Part model, mm, in its own coordinate system. Face numbers are marked on the shaded views. A direction names the side the tool comes from. Give positions to 0.01 mm unless a question says otherwise; leave off trailing zeros. Write each loop counter-clockwise with the first axis right and the second up, starting at its lowest first coordinate (ties: lowest second). Pieces come first, ordered by that corner, then holes.
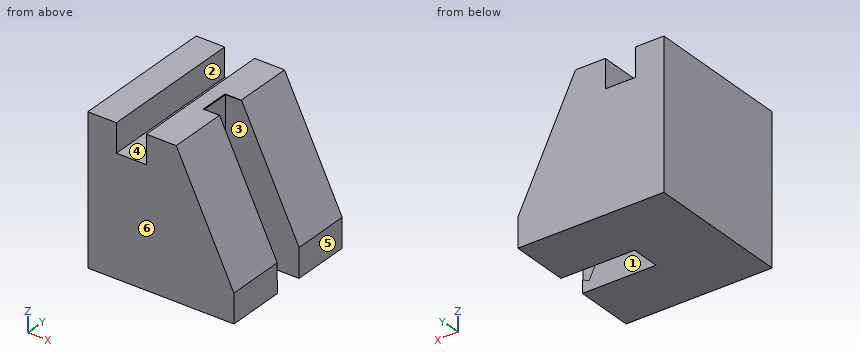
from build123d import *

# Parameters (mm, degrees)
F1_DEPTH = 100
F2_W     = 20
F2_H     = 89.6053736129
F3_DEPTH = 10
F4_DEPTH = 10
F5_DEPTH = 10
F6_W     = 50.2936672419
F6_H     = 19.8401175439
F7_DEPTH = 100


with BuildPart() as f1:
    # F0 (on Front) → F1 (new body)
    with BuildSketch(Plane.XZ):
        Polygon((-55.1563166082, 75.4929259419), (-74.7038125992, 75.4929259419), (-74.7038125992, -24.8185619712), (25.1119807363, -24.8185619712), (25.1119807363, -4.9872435629), (-14.2842791975, 75.4929259419), (-34.7202979028, 75.4929259419), (-34.7202979028, 55.9454262257), (-55.1563166082, 55.9454262257), align=None)
    extrude(amount=F1_DEPTH)

    # F2 (on face) → F3 (cut)
    with BuildSketch(Plane(origin=(18.2883118785, 0, 8.9524052067), x_dir=(0, 1, 0), z_dir=(0.8981623117, 0, 0.4396640329))):
        with Locations((-50, 29.2824978739)):
            Rectangle(F2_W, F2_H)
    extrude(amount=-F3_DEPTH, mode=Mode.SUBTRACT)

    # F4 (cut): a face of the model
    f4_faces = [f1.faces().sort_by_distance(p)[0] for p in [
        (-18.775090756, -50, 73.2946057774),
    ]]
    extrude(f4_faces, amount=-F4_DEPTH, mode=Mode.SUBTRACT)

    # F5 (cut): a face of the model
    f5_faces = [f1.faces().sort_by_distance(p)[0] for p in [
        (20.6211691778, -50, -7.1855637275),
    ]]
    extrude(f5_faces, amount=-F5_DEPTH, mode=Mode.SUBTRACT)

    # F6 (on face) → F7 (cut)
    with BuildSketch(Plane(origin=(0, 0, -24.8185619712), x_dir=(1, 0, 0), z_dir=(0, 0, -1))):
        with Locations((-0.0348528847, 49.7383717448)):
            Rectangle(F6_W, F6_H)
    extrude(amount=-F7_DEPTH, mode=Mode.SUBTRACT)


solid = f1.part
1) Drill centre lines: L1, parallel to Y at x = 15, z = -16.5; L2, parallel to Y at x = 13, z = 16.5; L3, parallel to Z at x = -50, y = -27. Where is each one in solid material? Low to high.
Check result:
L1: y = -100 to -59.66, -39.82 to 0
L2: y = -100 to -60, -39.82 to 0
L3: z = -24.82 to 55.95
2) Saw through at C-C (z = -1). Write the cut outline in (x, y).
Check result:
outline: (-74.7, -100) - (23.16, -100) - (23.16, -60) - (12.03, -60) - (12.03, -59.66) - (-25.18, -59.66) - (-25.18, -39.82) - (23.16, -39.82) - (23.16, 0) - (-74.7, 0) - close
3) Mould opens along X. For the marked faces 4, 5 and 6 say: +X half, -X half, draft (parallel to the pull), parting line (faces both ways), or undercut.
Check result:
face 4: undercut
face 5: +X half
face 6: draft
4) 3-axis set-ups, long thin cutter, end or side, ignore diameter. For the marked faces 1, 2 and 3: which of +Z, -Z, +X, -X, +Y, -Y reach the whole face in a straight line?
Check result:
face 1: +Z, -Z, +X
face 2: +Z, +Y, -Y
face 3: -Z, +X
5) Saw through at B-B (y = -9.5). Write the cut outline in (x, z), and give its area (3 significant figures).
Check result:
outline: (-74.7, -24.82) - (25.11, -24.82) - (25.11, -4.99) - (-14.28, 75.49) - (-34.72, 75.49) - (-34.72, 55.95) - (-55.16, 55.95) - (-55.16, 75.49) - (-74.7, 75.49) - close
area: 8,030 mm2
6) Saw through at A-A (x = -19.5). Write the cut outline in (y, z).
Check result:
outline: (-100, -24.82) - (-59.66, -24.82) - (-59.66, 63.4) - (-60, 63.4) - (-60, 75.49) - (-100, 75.49) - close; (-40, 75.18) - (-39.82, 75.18) - (-39.82, -24.82) - (0, -24.82) - (0, 75.49) - (-40, 75.49) - close
7) Saw through at D-D (x = -44). Write the cut outline in (y, z).
Check result:
outline: (-100, -24.82) - (0, -24.82) - (0, 55.95) - (-100, 55.95) - close
8) Flat gauge pins, fed straight in: P1, Ø10, axis at y = -51.5, z = 69.5, coming from the +X side; P2, Ø4, axis at x = 5, y = -63, coming from the +Z side. Where does each tip first touch, or does it go through?
Check result:
P1: stops at x = -25.18
P2: stops at z = 40.18
